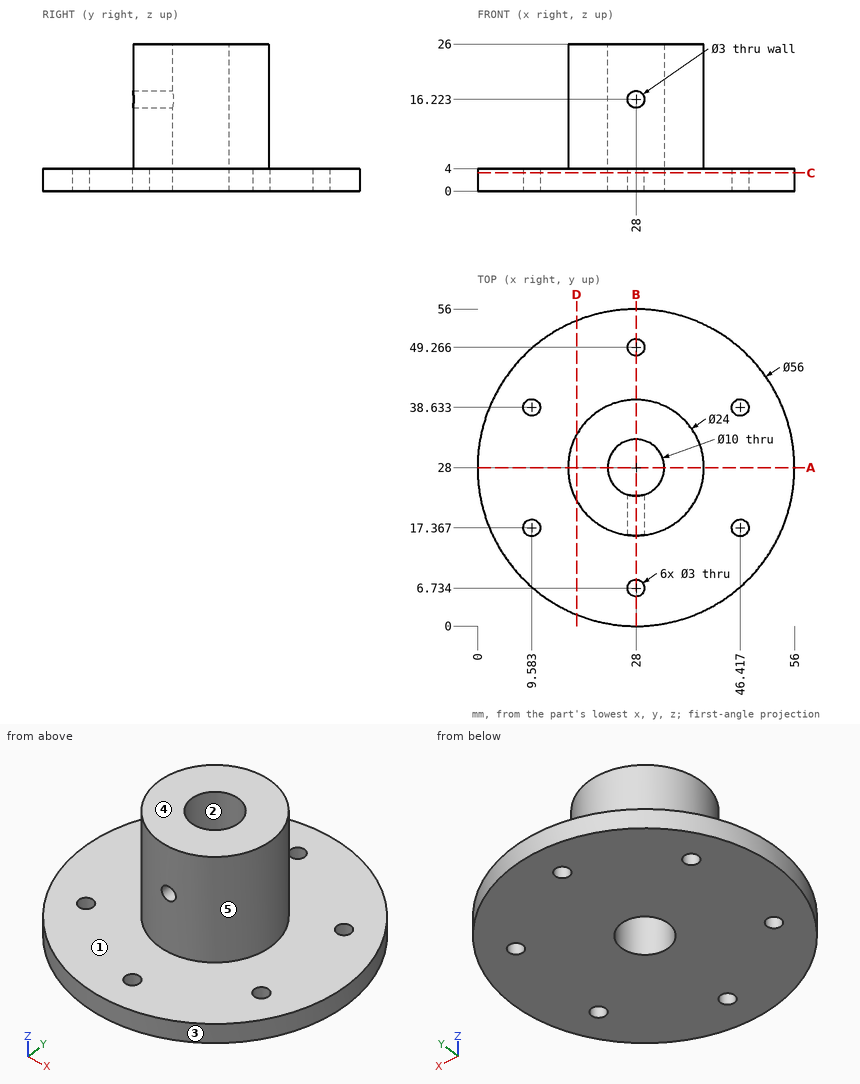
Could you check a few things on this drawing? It's one solid part, dimensions in mm from its lowest x, y, z. A direction names the side the tool comes from. Coordinates: 2 decimals unless noted, no trailing zeros. Order: outer loops, then holes, each group sorted by start corner. A loop starts at its lowest first (then second) coordinate and runs counter-clockwise, first axis right, second up.
1) Imagine slicing it at D-D on x = 17.5. List the corners of the cut face in (y, z) for me, and give its area (3 significant figures).
2) Imagine slicing it at C-C on z = 3.25. List the corners of the cut face in (x, y) for me (1 decimal).
3) Imagine slicing it at B-B on x = 28. List the corners of the cut face in (y, z) for me (1 decimal).
4) We'd pull the mould along Y, two halves only. Please class the marked faces 1, 2 and 3: +Y half, -Y half, draft (parallel to the pull), parting line (faces both ways), or undercut.
5) Will these pins go through, and if not, where does the flat tip stop? pin 1 (3.5 mm diameter, centred on x = 9.58, y = 38.63, fed in from +Z); pin 2 (5 mm diameter, centred on x = 28, z = 16.22, fed in from +Y); pin 3 (5 mm diameter, centred on x = 35, z = 21, fed in from -Y) (1 decimal).
6) Which directions (+Z, -Z, +X, -X, +Y, -Y) give clear straight access to the entire face, cutting with the end or side of a thin tool? Please do the marked faces 4 and 5.
7) Imagine slicing it at A-A on y = 28. List the corners of the cut face in (x, z) for me, and give its area (3 significant figures).
8) I need wall thicknesses on line 1 (Y direction, x = 28, z = 2.5) (1 decimal); line 2 (Y direction, x = 45.5, z = 3.5) (1 decimal); line 3 (Z direction, x = 28, y = 20). Which ranges of each line are inside material? Lowest first, please.
Response values:
1. outline: (2.04, 0) - (53.96, 0) - (53.96, 4) - (33.81, 4) - (33.81, 26) - (22.19, 26) - (22.19, 4) - (2.04, 4) - close
1. area: 463 mm2
2. outline: circle Ø56 at (28, 28); hole circle Ø3 at (9.6, 17.4); hole circle Ø3 at (9.6, 38.6); hole circle Ø10 at (28, 28); hole circle Ø3 at (28, 6.7); hole circle Ø3 at (28, 49.3); hole circle Ø3 at (46.4, 17.4); hole circle Ø3 at (46.4, 38.6)
3. outline: (0, 0) - (5.2, 0) - (5.2, 4) - (0, 4) - close; (8.2, 0) - (23, 0) - (23, 14.7) - (16, 14.7) - (16, 4) - (8.2, 4) - close; (16, 17.7) - (23, 17.7) - (23, 26) - (16, 26) - close; (33, 0) - (47.8, 0) - (47.8, 4) - (40, 4) - (40, 26) - (33, 26) - close; (50.8, 0) - (56, 0) - (56, 4) - (50.8, 4) - close
4. face 1: draft
4. face 2: undercut
4. face 3: parting line
5. pin 1: stops at z = 4
5. pin 2: stops at y = 40
5. pin 3: stops at y = 16.9
6. face 4: +Z, +X, -X, +Y, -Y
6. face 5: +Z
7. outline: (0, 0) - (23, 0) - (23, 26) - (16, 26) - (16, 4) - (0, 4) - close; (33, 0) - (56, 0) - (56, 4) - (40, 4) - (40, 26) - (33, 26) - close
7. area: 492 mm2
8. line 1: y = 0 to 5.2, 8.2 to 23, 33 to 47.8, 50.8 to 56
8. line 2: y = 6.1 to 16.2, 18.6 to 37.4, 39.8 to 49.9
8. line 3: z = 0 to 14.72, 17.72 to 26
